```python
from build123d import *

# Parameters (mm, degrees)
CUT_EXTRUDE3_DEPTH       = 50.352144442
CUT_EXTRUDE3_DEPTH_BACK  = 50.352144442
BOSS_EXTRUDE1_REACH      = 63.121
BOSS_EXTRUDE1_END_RADIUS = 18.415
SKETCH3_R                = 2.5146
FILLET1_R                = 0.762
CHAMFER1_SIZE            = 2.794
CHAMFER1_SIZE_2          = 2.888956472
FILLET3_R                = 2.54


with BuildPart() as part:
    # Sketch1 → Revolve1 (revolve)
    with BuildSketch(Plane.XY, mode=Mode.PRIVATE) as revolve1_sk:
        Polygon((-40.64, 13.7795), (0, 13.7795), (0, 16.383), (30.48, 16.383), (30.48, 17.653), (24.13, 18.415), (-7.62, 18.415), (-7.62, 16.256), (-19.3929, 15.875), (-19.3929, 19.0373), (-19.3929, 19.7993), (-22.098, 19.7993), (-24.384, 17.5133), (-27.94, 17.5133), (-27.94, 19.7231), (-32.234028859, 19.7231), (-34.544, 18.188619171), (-36.724705389, 16.007913782), (-40.64, 15.500375591), (-40.64, 14.732), align=None)
    revolve(revolve1_sk.sketch.rotate(Axis((-11.776127049, 0, 0), (1, 0, 0)), 90), axis=Axis((-11.776127049, 0, 0), (1, 0, 0)))

    # Sketch2 → Cut-Extrude3 (cut, two sides: drawn at the far end of the back side and taken through both)
    with BuildSketch(Plane.XY.offset(-CUT_EXTRUDE3_DEPTH_BACK)):
        with BuildLine():
            Line((13.882361942, 2.538487654), (30.48, 3.1115))
            Line((30.48, 3.1115), (30.48, -3.1115))
            Line((30.48, -3.1115), (13.882361942, -2.538487654))
            ThreePointArc((13.882361942, -2.538487654), (11.43, 0), (13.882361942, 2.538487654))
        make_face()
    extrude(amount=CUT_EXTRUDE3_DEPTH + CUT_EXTRUDE3_DEPTH_BACK, mode=Mode.SUBTRACT)

    # Boss-Extrude1: up to this cylinder (the profile starts outside it)
    boss_extrude1_end = Plane(origin=(11.938, 0, 0), z_dir=(-1, 0, 0)) * Cylinder(BOSS_EXTRUDE1_END_RADIUS, 164.072, mode=Mode.PRIVATE)
    # Sketch3 → Boss-Extrude1 (add, up to the surface)
    with BuildSketch(Plane(origin=(0, 21.336, 0), x_dir=(1, 0, 0), z_dir=(0, 1, 0)), mode=Mode.PRIVATE) as boss_extrude1_sk1:
        with Locations(Location((11.938, 0, 0), (0, 0, 270))):
            Circle(SKETCH3_R)
    boss_extrude1_tool1 = extrude(boss_extrude1_sk1.sketch, amount=-BOSS_EXTRUDE1_REACH, mode=Mode.PRIVATE) - boss_extrude1_end
    boss_extrude1 = boss_extrude1_tool1.solids().sort_by_distance((11.938, 21.336, 0))[0]
    add(boss_extrude1)

    # Mirror1: Boss-Extrude1 across plane
    add(boss_extrude1.mirror(Plane.ZX))

    # Fillet1
    fillet1_edges = [part.edges().sort_by_distance(p)[0] for p in [
        (-27.94, 0, -17.5133),
        (-19.3929, 0, -15.875),
    ]]
    fillet(fillet1_edges, radius=FILLET1_R)

    # Chamfer1
    # the kernel refuses this chamfer: 2.888956472, 2.794 mm, written as the material it adds along each edge
    with BuildSketch(Plane(origin=(0, 0, 0), x_dir=(0, 0, 1), z_dir=(0, 1, 0))) as chamfer1_piece_1_section:
        Polygon((16.383 - CHAMFER1_SIZE, 0), (16.383, CHAMFER1_SIZE), (16.383, 0), align=None)
    chamfer1_piece_1 = revolve(axis=Axis((0, 0, 0), (1, 0, 0)), mode=Mode.PRIVATE)
    chamfer1_piece_1 = chamfer1_piece_1 - Plane(origin=(1.479100002, 0, 0), x_dir=(0, 0, 1), z_dir=(1, 0, 0)) * Cylinder(13.7795, 66, mode=Mode.PRIVATE)
    add(chamfer1_piece_1)
    with BuildSketch(Plane(origin=(-7.62, 0, 0), x_dir=(0, 0, 1), z_dir=(0, 1, 0))) as chamfer1_piece_2_section:
        Polygon((16.256 - CHAMFER1_SIZE_2 * 0.0323455257839, -CHAMFER1_SIZE_2 * 0.999476746721), (16.256 + CHAMFER1_SIZE, 0), (16.256, 0), align=None)
    chamfer1_piece_2 = revolve(axis=Axis((-7.62, 0, 0), (1, 0, 0)), mode=Mode.PRIVATE)
    chamfer1_piece_2 = chamfer1_piece_2 & Plane(origin=(-9.368047324, 0, 0), x_dir=(0, 0, 1), z_dir=(-1, 0, 0)) * Cylinder(18.415, 77, mode=Mode.PRIVATE)
    add(chamfer1_piece_2)

    # Fillet3
    fillet3_edges = [part.edges().sort_by_distance(p)[0] for p in [
        (-10.507444816, 0, -16.162555184),
        (2.794, 0, -16.383),
        (-8.255, 0, -18.415),
        (0.1905, 0, -13.7795),
    ]]
    fillet(fillet3_edges, radius=FILLET3_R)


solid = part.part
```
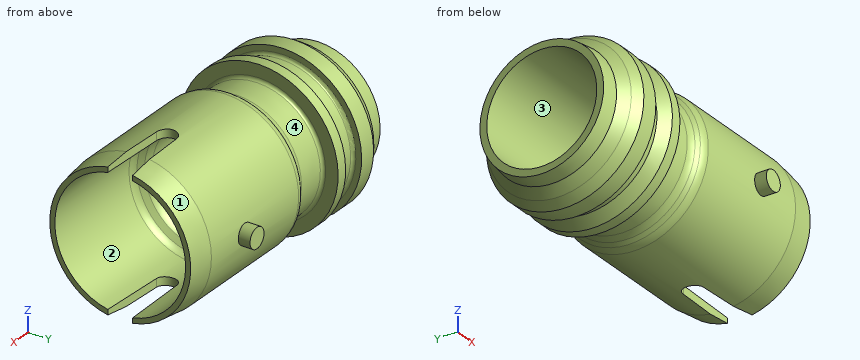
Check sheet for the modelled part. Datum: model origin and axes. Units: mm. Face numbers are marked on the shaded views. A direction names the side the tool comes from. Give positions to 0.01 mm unless a question says otherwise; leave off trailing zeros. Use CSV: the item, a comma, the result in double quotes. Start each with the question number.
Q1. Scan lines: line 1 along Z through (x, y) = (8.5, 2.5); line 2 along X through (y, z) = (-19, -1); line 3 along Y through (x, z) = (-21, 0). Record each from-to range of solid material in increasing order.
Q2. Release check for a two-part mould opening along Z. For the marked faces 1 and 2 record: +Z half, -Z half, draft (parallel to the pull), parting line (faces both ways), or undercut.
Q3. Tool access check on the marked faces 3 and 4. Record the directions out of +Z, -Z, +X, -X, +Y, -Y that give a thin tool (end or side, any length) a straight path to the whole face; none if there is none.
Q4. Depth check by flat-ended pin: P1, Ø8, axis at x = 20, y = -6.5, coming from the +Z side; P2, Ø5, axis at x = -32, z = 6.5, coming from the -Y side; P3, Ø6, axis at x = -12.5, y = -14, coming from the +Z side. Enter the tip coordinate at first touch or a pass-through.
Working result:
1,line 1,"z = -18.24 to -16.19, 16.19 to 18.24"
1,line 2,"x = -33.28 to -27.94, -22.87 to -19.39, 9.63 to 14.25"
1,line 3,"y = -19.8 to -13.78, 13.78 to 19.8"
2,face 1,"parting line"
2,face 2,"undercut"
3,face 3,"+X, -X"
3,face 4,"none"
4,P1,"stops at z = 18.22"
4,P2,"stops at y = -19.31"
4,P3,"stops at z = 11.76"
